Geometry: see drawing. Coordinates: mm, zero at the bounding-box minimum. A direction names the side the tool comes from. Give positions to 0.01 mm unless a question says otherwise; leave off trailing zeros. Loops run counter-clockwise (first coordinate to the right, second up) from the corner with the lowest first, then second, coordinate; pieces in that order, holes last. Notation, with made-up numbers: (16.5, 62) - (28.5, 62) arc R13 cw to (28.5, 71) - close; hole circle Ø10 at (5, 21). An arc over 180 degrees is marked (long way). Use one line per item in the form item = value.
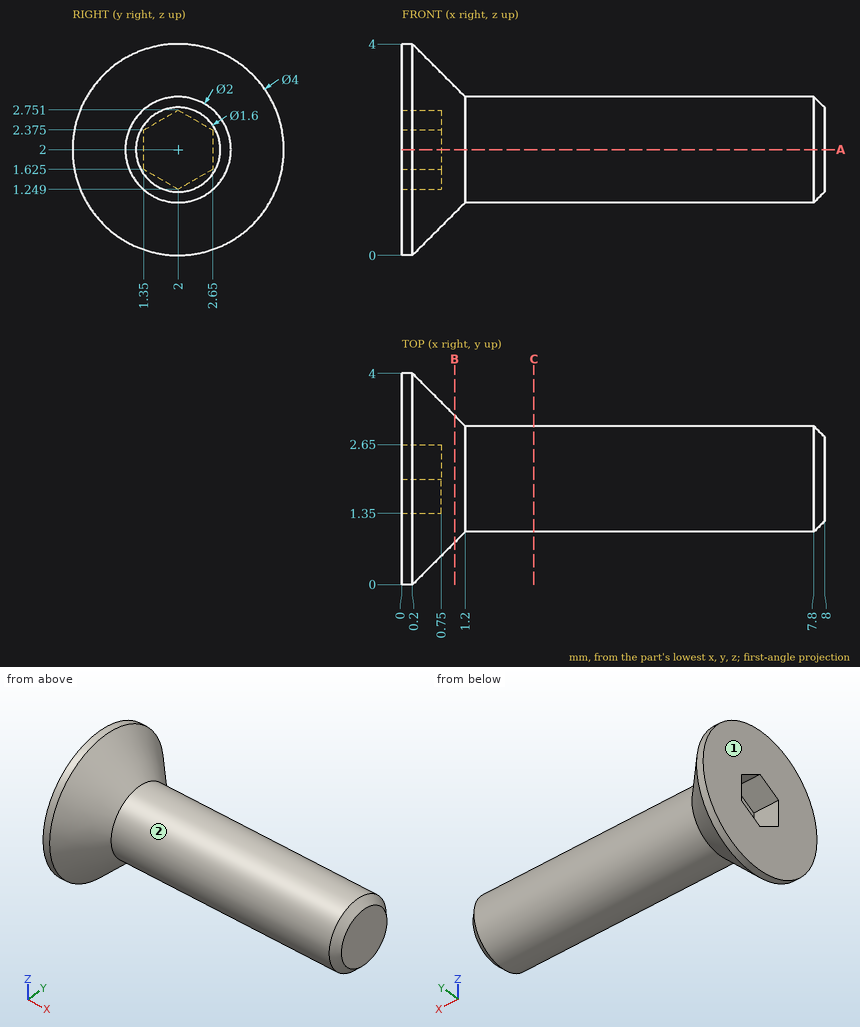
(1) Access query for the marked faces 1 and 2. Directions: +Z, -Z, +X, -X, +Y, -Y. A direction counts if a zero-diameter tool reaches every point of the face in a straight line with its end or side. Return the directions, or none.
Solution:
face_1 = +Z, -Z, -X, +Y, -Y
face_2 = +X
(2) Cut plane A-A (z = 2). Return the cut outline in (x, y), plus the area to 3 significant figures.
Solution:
outline = (0, 0) - (0.2, 0) - (1.2, 1) - (7.8, 1) - (8, 1.2) - (8, 2.8) - (7.8, 3) - (1.2, 3) - (0.2, 4) - (0, 4) - (0, 2.65) - (0.75, 2.65) - (0.75, 1.35) - (0, 1.35) - close
area = 16.4 mm2
(3) Cut plane B-B (x = 1). Return the cut outline in (y, z).
Solution:
outline = circle Ø2.4 at (2, 2)
(4) Cut plane C-C (x = 2.5). Return the cut outline in (y, z).
Solution:
outline = circle Ø2 at (2, 2)
(5) Material intervals for L1, parallel to Z at x = 6, y = 2; L2, parallel to X at y = 2.6, z = 1.95; L3, parallel to X at y = 0.6, z = 2.45, sorted ascending. Write a range as from..to.
Solution:
L1 = 1..3
L2 = 0.75..8
L3 = 0..0.73
(6) Pin query (flat end, axial travel): P1, Ø1, axis at x = 2, y = 1.5, coming from the -Z side; P2, Ø2, axis at x = 3.5, z = 1, coming from the -Y side; P3, Ø2, axis at x = 4, z = 1, coming from the +Y side. Return the tip coordinate at first contact, or that it passes through.
Solution:
P1 = 1
P2 = 1
P3 = 3
